```python
from build123d import *

# Parameters (mm, degrees)
SKETCH_R     = 1.8
PAD_DEPTH    = 3
SKETCH001_W  = 42
SKETCH001_H  = 2
PAD001_DEPTH = 3


with BuildPart() as part:
    # Sketch → Pad (new body)
    with BuildSketch(Plane.XY):
        Polygon((-21, 21), (21, 21), (21, -21), (0, -21), (-21, -21), (-21, 0), align=None)
        with Locations((0, 12.5)):
            Circle(SKETCH_R, mode=Mode.SUBTRACT)
        with Locations((10.825318, 6.25)):
            Circle(SKETCH_R, mode=Mode.SUBTRACT)
        with Locations((10.825318, -6.25)):
            Circle(SKETCH_R, mode=Mode.SUBTRACT)
        with Locations((0, -12.5)):
            Circle(SKETCH_R, mode=Mode.SUBTRACT)
        with Locations((-10.825318, -6.25)):
            Circle(SKETCH_R, mode=Mode.SUBTRACT)
        with Locations((-10.825318, 6.25)):
            Circle(SKETCH_R, mode=Mode.SUBTRACT)
        Circle(SKETCH_R, mode=Mode.SUBTRACT)
    extrude(amount=PAD_DEPTH)

    # Sketch001 → Pad001 (new body)
    with BuildSketch(Plane.XY.offset(3)):
        Polygon((-21, 21), (21, 21), (21, 19), (0, 19), (-21, 19), align=None)
        with Locations((0, -20)):
            Rectangle(SKETCH001_W, SKETCH001_H)
    extrude(amount=PAD001_DEPTH)


solid = part.part
```
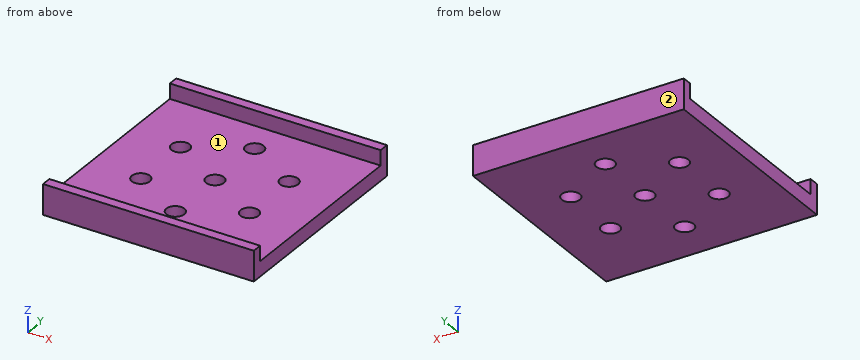
Work out the finished part from the listing and answer in its coordinate system (mm). Face numbers are marked on the shaded views. A direction names the side the tool comes from. Round coordinates to 2 decimals unless told otherwise and drop trailing zeros. Loops run counter-clockwise (first coordinate to the right, second up) from the corner with the lowest first, then second, coordinate; pieces in that order, holes last. Notation, with made-up numbers: M 3.5,-29.75 L 45.5,-29.75 A10 ccw 45.5,-10.75 Z; hole C 17,28 d7. An arc over 180 degrees is marked long. Use CSV: the item, a comma, the result in double quotes.
Q1. Section D-D, the plane y = -12.5 is taken. Determine the outline of the cut face in (x, z), then the cut area to 3 significant figures.
Determined:
outline,"M -21,0 L -1.8,0 L -1.8,3 L -21,3 Z; M 1.8,0 L 21,0 L 21,3 L 1.8,3 Z"
area,"115 mm2"
Q2. Each of these flat-tipped pins is pushed along its axis until it touches: pin 1 (6 mm diameter, centred on x = 0, y = 12.5, fed in from +Z); pin 2 (3 mm diameter, centred on x = 10.83, y = -6.25, fed in from +Z). Where does it stop, or does it pass through?
Determined:
pin 1,"z = 3"
pin 2,"through"
Q3. Section B-B, the plane y = -6.25 is taken. Determine the outline of the cut face in (x, z).
Determined:
outline,"M -21,0 L -12.63,0 L -12.63,3 L -21,3 Z; M -9.03,0 L 9.03,0 L 9.03,3 L -9.03,3 Z; M 12.63,0 L 21,0 L 21,3 L 12.63,3 Z"
Q4. A tool of negligible diameter and unlimited length cuts with its end or side. For the marked faces 1 and 2, from which of +Z, -Z, +X, -X, +Y, -Y can it reach the whole face along a straight path? Write none if from no direction.
Determined:
face 1,"+Z, +X, -X"
face 2,"+Z, -Z, +X, -X, +Y"
Q5. Consider L1, parallel to Y at x = 0, z = 2.45; L2, parallel to Y at x = 3, z = 3.7; L3, parallel to Y at x = 11.5, z = 1.95. Determine where each line is inside the solid, lowest interval first.
Determined:
L1,"-21 to -14.3, -10.7 to -1.8, 1.8 to 10.7, 14.3 to 21"
L2,"-21 to -19, 19 to 21"
L3,"-21 to -7.92, -4.58 to 4.58, 7.92 to 21"
Q6. Section A-A, the plane x = 0 is taken. Determine the outline of the cut face in (y, z).
Determined:
outline,"M -21,0 L -14.3,0 L -14.3,3 L -19,3 L -19,6 L -21,6 Z; M -10.7,0 L -1.8,0 L -1.8,3 L -10.7,3 Z; M 1.8,0 L 10.7,0 L 10.7,3 L 1.8,3 Z; M 14.3,0 L 21,0 L 21,6 L 19,6 L 19,3 L 14.3,3 Z"
Q7. Section C-C, the plane z = 2.2 is taken. Determine the outline of the cut face in (x, y), then the cut area to 3 significant figures.
Determined:
outline,"M -21,-21 L 21,-21 L 21,21 L -21,21 Z; hole C -10.83,-6.25 d3.6; hole C -10.83,6.25 d3.6; hole C 0,-12.5 d3.6; hole C 0,0 d3.6; hole C 0,12.5 d3.6; hole C 10.83,-6.25 d3.6; hole C 10.83,6.25 d3.6"
area,"1,690 mm2"
